Check sheet for the modelled part. Datum: model origin and axes. Units: mm. A direction names the side the tool comes from. Give positions to 0.01 mm unless a question says otherwise; leave off trailing zeros. Write each loop counter-clockwise with the first axis right and the second up, starting at its lowest first coordinate (ties: lowest second). Pieces come first, ordered by that corner, then holes. Notation, with made-up numbers: (-31.75, 34) - (-7.75, 34) arc R23 ccw to (-7.75, 45) - close; hole circle Ø5 at (21, 4). An arc over 180 degrees is marked (long way). Return JSON: item names as keys, results as strings. Group by question number.
```python
from build123d import *

# Parameters (mm, degrees)
SKETCH1_W           = 133.35
SKETCH1_H           = 38.1
BOSS_EXTRUDE1_DEPTH = 3.175
SKETCH2_W           = 3.2258
SKETCH2_H           = 6.35
BOSS_EXTRUDE2_DEPTH = 3.175


with BuildPart() as part:
    # Sketch1 → Boss-Extrude1 (new body)
    with BuildSketch(Plane(origin=(0, 0, 0), x_dir=(0, 0, -1), z_dir=(1, 0, 0))):
        Rectangle(SKETCH1_W, SKETCH1_H)
    extrude(amount=BOSS_EXTRUDE1_DEPTH)

    # Sketch2 → Boss-Extrude2 (add)
    with BuildSketch(Plane.ZY):
        with Locations((-68.2879, 8.255)):
            Rectangle(SKETCH2_W, SKETCH2_H)
        with Locations((-68.2879, -10.795)):
            Rectangle(SKETCH2_W, SKETCH2_H)
    boss_extrude2 = extrude(amount=-BOSS_EXTRUDE2_DEPTH)

    # Mirror1: Boss-Extrude2 across plane
    add(boss_extrude2.mirror(Plane.XY))


solid = part.part
```
Item 1: Material ranges on line 1 along Z through (x, y) = (0.3, -7) (3 decimals), recorded low to high. Write a range as from..to.
Item 2: Depth check by flat-ended pin: pin 1 (1.6 mm diameter, centred on x = 1.5, y = 16, fed in from +Z) (3 decimals); pin 2 (1.6 mm diameter, centred on x = 2.5, y = -16.5, fed in from -Z) (3 decimals); pin 3 (1 mm diameter, centred on x = 1.5, z = -67.5, fed in from +Y). Enter the tip coordinate at first touch or a pass-through.
Item 3: Section check A-A on x = 2.5. Record the cut outline in (y, z) (3 decimals).
Item 4: Section check B-B on y = -4. Record the cut outline in (x, z) (3 decimals).
Item 5: Mould release check, pull along Y, two halves, no side actions. Record for faces 1 (the face through (2, -7.62, -68)), 2 (the face through (2, 5.08, -68)), 3 (the face through (2, -13.97, -68)), 4 (the face through (3.175, 0, 1)): +Y half, -Y half, draft (parallel to the pull), parting line (faces both ways), or undercut.
Item 6: Access from +Z, -Z, +X, -X, +Y, -Y to the whole of each face (thin tool, end or side, straight path). Record for faces 5 (the face through (2, 5.08, 68)), 6 (the face through (2, 11.43, 68)), 7 (the face through (2, -17, 66.675)).
Reply:
{
 "1": {"line 1": "-66.675..66.675"},
 "2": {"pin 1": "z = 66.675", "pin 2": "z = -66.675", "pin 3": "y = 11.43"},
 "3": {"outline": "(-19.05, -66.675) - (-13.97, -66.675) - (-13.97, -69.901) - (-7.62, -69.901) - (-7.62, -66.675) - (5.08, -66.675) - (5.08, -69.901) - (11.43, -69.901) - (11.43, -66.675) - (19.05, -66.675) - (19.05, 66.675) - (11.43, 66.675) - (11.43, 69.901) - (5.08, 69.901) - (5.08, 66.675) - (-7.62, 66.675) - (-7.62, 69.901) - (-13.97, 69.901) - (-13.97, 66.675) - (-19.05, 66.675) - close"},
 "4": {"outline": "(0, -66.675) - (3.175, -66.675) - (3.175, 66.675) - (0, 66.675) - close"},
 "5": {"face 1": "undercut", "face 2": "undercut", "face 3": "-Y half", "face 4": "draft"},
 "6": {"face 5": "+Z, +X, -X", "face 6": "+Z, +X, -X, +Y", "face 7": "+Z, +X, -X, -Y"}
}
